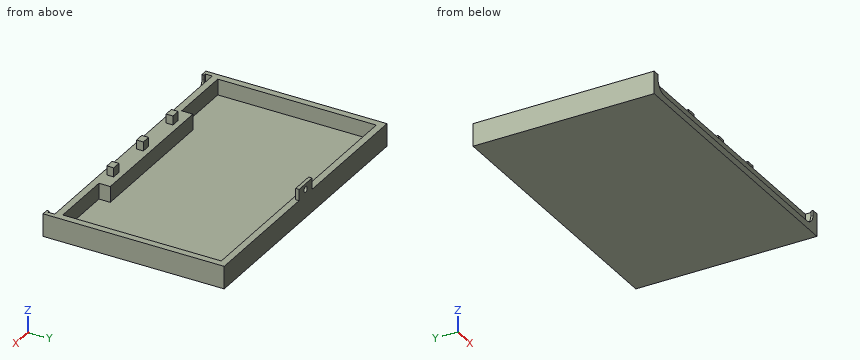
```python
from build123d import *

# Parameters (mm, degrees)
F0_W      = 125
F0_H      = 80
F1_DEPTH  = 10
F3_DEPTH  = 7
F4_W      = 10
F4_H      = 1.5
F5_DEPTH  = 5
F6_R      = 1.25
F7_DEPTH  = 25
F8_W      = 4
F8_H      = 3
F9_DEPTH  = 4
F11_DEPTH = 4
F12_W     = 121
F12_H     = 3
F13_DEPTH = 8


with BuildPart() as f1:
    # F0 (on Top) → F1 (new body)
    with BuildSketch(Plane.XY):
        Rectangle(F0_W, F0_H)
    extrude(amount=F1_DEPTH)

    # F2 (on face) → F3 (cut)
    with BuildSketch(Plane.XY.offset(10)):
        Polygon((59.5, 37), (-59.5, 37), (-59.5, -33), (-31.725, -33), (-31.725, -28), (31.725, -28), (31.725, -33), (59.5, -33), align=None)
    extrude(amount=-F3_DEPTH, mode=Mode.SUBTRACT)

    # F4 (on face) → F5 (join)
    with BuildSketch(Plane.XY.offset(10)):
        with Locations((0, 39.25)):
            Rectangle(F4_W, F4_H)
    extrude(amount=F5_DEPTH)

    # F6 (on face) → F7 (cut)
    with BuildSketch(Plane(origin=(0, 40, 0), x_dir=(-1, 0, 0), z_dir=(0, 1, 0))):
        with Locations((0, 12.5)):
            Circle(F6_R)
    extrude(amount=-F7_DEPTH, mode=Mode.SUBTRACT)

    # F8 (on face) → F9 (join)
    with BuildSketch(Plane.XY.offset(10)):
        with Locations((0, -32)):
            Rectangle(F8_W, F8_H)
        with Locations((22.725, -32)):
            Rectangle(F8_W, F8_H)
        with Locations((-22.725, -32)):
            Rectangle(F8_W, F8_H)
    extrude(amount=F9_DEPTH)

    # F10 (on face) → F11 (cut)
    with BuildSketch(Plane.XZ.offset(40)):
        with BuildLine():
            ThreePointArc((54.551, 3), (58.050471, 4.449529), (59.5, 7.949))
            Line((59.5, 7.949), (59.5, 10))
            Line((59.5, 10), (0, 10))
            Line((0, 10), (-59.5, 10))
            Line((-59.5, 10), (-59.5, 7.949))
            ThreePointArc((-59.5, 7.949), (-58.050471, 4.449529), (-54.551, 3))
            Line((-54.551, 3), (0, 3))
            Line((0, 3), (54.551, 3))
        make_face()
    extrude(amount=-F11_DEPTH, mode=Mode.SUBTRACT)

    # F12 (on face) → F13 (cut)
    with BuildSketch(Plane.XY.offset(10)):
        with Locations((0, -37.5)):
            Rectangle(F12_W, F12_H)
    extrude(amount=-F13_DEPTH, mode=Mode.SUBTRACT)


solid = f1.part
```
The model under review builds one solid part; all positions refer to its coordinate system, in mm. Coordinates: 2 decimals unless noted, no trailing zeros. Order: outer loops, then holes, each group sorted by start corner. A loop starts at its lowest first (then second) coordinate and runs counter-clockwise, first axis right, second up. Notation, with made-up numbers: (-10, 39) -> (44, 39) arc R14 cw to (44, 45) -> close; hole circle Ø8 at (24.25, 14). An arc over 180 degrees is marked (long way). Answer in a Markdown table with one row per item. Add a question column.
Item 1: Clearance check with flat-ended pins moving along their axes: pin 1 (6 mm diameter, centred on x = -16, y = -5.5, fed in from -Z); pin 2 (0.9 mm diameter, centred on x = -22.5, y = -31.5, fed in from +Z); pin 3 (0.5 mm diameter, centred on x = -13, y = -39.5, fed in from +Z); pin 4 (2.5 mm diameter, centred on y = -32, z = 11.5, fed in from +X) (3 decimals). State where each tip first meets the part, or that it passes through.
Item 2: We need section A-A on x = 0. Write out the cut boundary in (y, z).
Item 3: We need section D-D on x = 36.5. Write out the cut boundary in (y, z).
Item 4: To check wall thickness, follow probe 1 along Y at (x, z) = (-38.5, 4); probe 2 along X at (y, z) = (-13.5, 6.25); probe 3 along Y at (x, z) = (-9, 7.5). State the ranges of each line that lie inside material, in increasing order.
Item 5: We need section C-C on y = 31. Write out the cut boundary in (x, z), plus the area to 3 significant figures.
Item 6: We need section B-B on z = 12.5. Write out the cut boundary in (x, y) (3 decimals), plus the area to 4 significant figures.
Final values:
| question | item | result |
|---|---|---|
| 1 | pin 1 | stops at z = 0 |
| 1 | pin 2 | stops at z = 14 |
| 1 | pin 3 | stops at z = 3 |
| 1 | pin 4 | stops at x = 24.725 |
| 2 | outline | (-40, 0) -> (40, 0) -> (40, 11.25) -> (38.5, 11.25) -> (38.5, 10) -> (37, 10) -> (37, 3) -> (-28, 3) -> (-28, 10) -> (-30.5, 10) -> (-30.5, 14) -> (-33.5, 14) -> (-33.5, 10) -> (-36, 10) -> (-36, 2) -> (-39, 2) -> (-39, 3) -> (-40, 3) -> close; (38.5, 13.75) -> (40, 13.75) -> (40, 15) -> (38.5, 15) -> close |
| 3 | outline | (-40, 0) -> (40, 0) -> (40, 10) -> (37, 10) -> (37, 3) -> (-33, 3) -> (-33, 10) -> (-36, 10) -> (-36, 2) -> (-39, 2) -> (-39, 3) -> (-40, 3) -> close |
| 4 | probe 1 | y = -36 to -33, 37 to 40 |
| 4 | probe 2 | x = -62.5 to -59.5, 59.5 to 62.5 |
| 4 | probe 3 | y = -36 to -28, 37 to 40 |
| 5 | outline | (-62.5, 0) -> (62.5, 0) -> (62.5, 10) -> (59.5, 10) -> (59.5, 3) -> (-59.5, 3) -> (-59.5, 10) -> (-62.5, 10) -> close |
| 5 | area | 417 mm2 |
| 6 | outline | (-24.725, -33.5) -> (-20.725, -33.5) -> (-20.725, -30.5) -> (-24.725, -30.5) -> close; (-5, 38.5) -> (-1.25, 38.5) -> (-1.25, 40) -> (-5, 40) -> close; (-2, -33.5) -> (2, -33.5) -> (2, -30.5) -> (-2, -30.5) -> close; (1.25, 38.5) -> (5, 38.5) -> (5, 40) -> (1.25, 40) -> close; (20.725, -33.5) -> (24.725, -33.5) -> (24.725, -30.5) -> (20.725, -30.5) -> close |
| 6 | area | 47.25 mm2 |
